Part model, mm, in its own coordinate system. A direction names the side the tool comes from. Round coordinates to 2 decimals unless told otherwise and drop trailing zeros. Loops run counter-clockwise (first coordinate to the right, second up) from the corner with the lowest first, then second, coordinate; pieces in that order, holes last. Notation, with made-up numbers: (89, 11.25) - (131, 11.25) arc R22 ccw to (131, 23.25) - close; hole circle Ø11 at (42.25, -26). An arc over 180 degrees is marked (long way). Write each question's results on one line, items separated by ' | '. Start each with the question number.
(1) Cut at C-C, the plane x = 47.5. List the corners of the cut face in (y, z), then the cut area to 3 significant figures.
(2) Cut at B-B, the plane z = 45. List the corners of the cut face in (x, y).
(3) Flat gauge pins, fed straight in: P1, Ø3, axis at y = 1.5, z = 42.5, coming from the -X side; P2, Ø3, axis at x = 49, y = 4, coming from the -Z side. Where does each tip first touch, or does it go through?
(4) Cut at D-D, the plane z = 49.5. List the corners of the cut face in (x, y), then the cut area to 3 significant figures.
(5) Mould opens along X. For faces 3 (the face through (71.77, 3, 48)), 4 (the face through (20, 3, 45.869)), 5 (the face through (46, 3, 45.869)), 6 (the face through (39.939, 3, 43)) say: released by +X, released by -X, zero draft, split by the parting line, or undercut.
(6) Tool access for faces 1 (the face through (14.399, 3.131, 50.196)), 2 (the face through (33.59, 3, 43)): list every direction of +Z, -Z, +X, -X, +Y, -Y with a clear straight run to the whole face (end or side of a thin tool).
(7) Drill centre lines: L1, parallel to Z at x = 44, y = 5.5; L2, parallel to X at y = 3.5, z = 42.75; L3, parallel to X at y = 1, z = 40.5. Where is each one in solid material? Low to high.
from build123d import *

# Parameters (mm, degrees)
BOSS_EXTRUDE1_DEPTH = 6.35
FILLET1_R           = 1.5875
FILLET2_R           = 6.35
FILLET3_R           = 3.175
SKETCH2_W           = 6.35
SKETCH2_H           = 6.35
BOSS_EXTRUDE2_DEPTH = 6.35


with BuildPart() as part:
    # Sketch1 → Boss-Extrude1 (new body)
    with BuildSketch(Plane(origin=(0, 0, 0), x_dir=(1, 0, 0), z_dir=(0, 1, 0))):
        with BuildLine():
            Line((52.558738922, -45.868730992), (33.5895, -45.868730992))
            Line((33.5895, -45.868730992), (6.2845, -45.868730992))
            Line((6.2845, -45.868730992), (24.145239996, -55.393730992))
            Line((24.145239996, -55.393730992), (71.770239996, -55.393730992))
            Line((71.770239996, -55.393730992), (71.770239996, -34.743530992))
            ThreePointArc((71.770239996, -34.743530992), (65.371223106, -45.84366442), (52.558738922, -45.868730992))
        make_face()
    extrude(amount=BOSS_EXTRUDE1_DEPTH)

    # Fillet1
    fillet1_edges = [part.edges().sort_by_distance(p)[0] for p in [
        (71.770239996, 3.175, 34.743530992),
        (52.558738922, 3.175, 45.868730992),
    ]]
    fillet(fillet1_edges, radius=FILLET1_R)

    # Fillet2
    fillet2_edges = [part.edges().sort_by_distance(p)[0] for p in [
        (24.145239996, 3.175, 55.393730992),
    ]]
    fillet(fillet2_edges, radius=FILLET2_R)

    # Fillet3
    fillet3_edges = [part.edges().sort_by_distance(p)[0] for p in [
        (71.770239996, 3.175, 55.393730992),
    ]]
    fillet(fillet3_edges, radius=FILLET3_R)

    # Sketch2 → Boss-Extrude2 (add)
    with BuildSketch(Plane(origin=(0, 0, 45.868730992), x_dir=(-1, 0, 0), z_dir=(0, 0, -1))):
        with Locations((-36.7645, 3.175)):
            Rectangle(SKETCH2_W, SKETCH2_H)
    extrude(amount=BOSS_EXTRUDE2_DEPTH)


solid = part.part
A:
1) outline: (0, 45.87) - (6.35, 45.87) - (6.35, 55.39) - (0, 55.39) - close | area: 60.5 mm2
2) outline: (33.59, 0) - (39.94, 0) - (39.94, 6.35) - (33.59, 6.35) - close; (66.65, 0) - (71.77, 0) - (71.77, 6.35) - (66.65, 6.35) - close
3) P1: x = 33.59 | P2: z = 45.87
4) outline: (13.09, 0) - (71.77, 0) - (71.77, 6.35) - (13.09, 6.35) - close | area: 373 mm2
5) face 3: released by +X | face 4: zero draft | face 5: undercut | face 6: undercut
6) face 1: +Z, -X, +Y, -Y | face 2: -Z, -X, +Y, -Y
7) L1: 45.87 to 55.39 | L2: 33.59 to 39.94, 68.97 to 71.4 | L3: 33.59 to 39.94
